Could you check a few things on this model? Use its own coordinates, in mm. Give positions to 0.01 mm unless a question says otherwise; leave off trailing zeros. Order: outer loops, then holes, each group sorted by start corner. A loop starts at its lowest first (then second) coordinate and runs counter-clockwise, first axis right, second up. Notation, with made-up numbers: (83.25, 77.25) -> (115.25, 77.25) arc R25 ccw to (115.25, 107.25) -> close; hole circle Ø5 at (33, 10.25). An arc over 180 degrees is marked (long way). Answer as CSV lines item,"result". Start each with the question number.
(1) I want a section at A-A (x = 0). Please give me the cut outline in (y, z), plus the area to 3 significant figures.
(2) I need wall thicknesses on L1, parallel to Y at x = 0.25, z = 3.25; L2, parallel to X at y = -55, z = 1.75; L3, parallel to Y at x = -1.25, z = -2. Which ranges of each line are inside material? Lowest first, please.
(3) I want a section at C-C (y = -14). Please give me the cut outline in (x, z), plus the area to 3 significant figures.
(4) I want a section at B-B (y = 62.5). Please give me the cut outline in (x, z).
(5) Will these pins go through, and if not, where does the flat tip stop? pin 1 Ø1.4 at (y, z) = (78, 0) entering from -X; pin 2 Ø3 at (y, z) = (38.5, 0) entering from -X; pin 3 Ø1 at (x, y) = (-3, -3) entering from -Z.
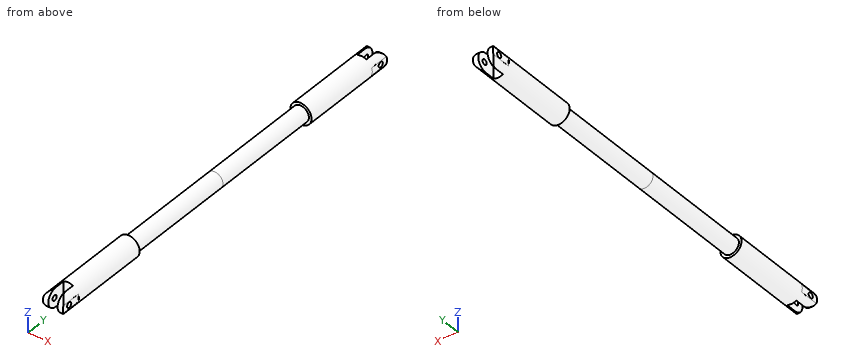
```python
from build123d import *

# Parameters (mm, degrees)
SKETCH2_W               = 3.5
SKETCH2_H               = 22
SKETCH2_W_2             = 3.489149722
SKETCH2_H_2             = 10.808558849
SKETCH2_W_3             = 5.104041679
SKETCH2_H_3             = 8.66936491
CUT_EXTRUDE1_DEPTH      = 10
SKETCH3_R               = 1
CUT_EXTRUDE2_DEPTH      = 1.25
CUT_EXTRUDE2_DEPTH_BACK = 8.75
CUT_EXTRUDE3_DEPTH      = 1.25
CUT_EXTRUDE3_DEPTH_BACK = 8.75


with BuildPart() as part:
    # Sketch1 → Revolve1 (revolve)
    with BuildSketch(Plane.XY, mode=Mode.PRIVATE) as revolve1_sk:
        Polygon((0, -75), (0, 75), (-3, 75), (-3, -35), (-4, -35), (-4, -75), align=None)
    revolve(revolve1_sk.sketch.rotate(Axis((0, -75, 0), (0, 1, 0)), 180), axis=Axis((0, -75, 0), (0, 1, 0)))  # turned: the seam where the file's is

    # Sketch2 → Cut-Extrude1 (cut, symmetric)
    with BuildSketch(Plane.XY):
        with Locations((0, -75)):
            Rectangle(SKETCH2_W, SKETCH2_H)
        with Locations((-5.494574861, -69.404279425)):
            Rectangle(SKETCH2_W_2, SKETCH2_H_2)
        with Locations((6.302020839, -68.334682455)):
            Rectangle(SKETCH2_W_3, SKETCH2_H_3)
    extrude(amount=CUT_EXTRUDE1_DEPTH, both=True, mode=Mode.SUBTRACT)

    # Sketch3 → Cut-Extrude2 (cut, two sides)
    with BuildSketch(Plane(origin=(3.75, 0, 0), x_dir=(0, 0, -1), z_dir=(1, 0, 0))) as cut_extrude2_sk:
        with Locations(Location((0, -68.334682455, 0), (0, 0, 90))):  # turned: the seam where the file's is
            Circle(SKETCH3_R)
    extrude(amount=CUT_EXTRUDE2_DEPTH, mode=Mode.SUBTRACT)
    extrude(cut_extrude2_sk.sketch, amount=-CUT_EXTRUDE2_DEPTH_BACK, mode=Mode.SUBTRACT)

    # Sketch4 → Cut-Extrude3 (cut, two sides)
    with BuildSketch(Plane(origin=(3.75, 0, 0), x_dir=(0, 0, -1), z_dir=(1, 0, 0))) as cut_extrude3_sk:
        with BuildLine():
            Line((-3.596873642, -67.828802158), (-5.675638146, -67.828802158))
            Line((-5.675638146, -67.828802158), (-5.675638146, -76.926900892))
            Line((-5.675638146, -76.926900892), (6.407188639, -76.926900892))
            Line((6.407188639, -76.926900892), (6.407188639, -67.828802158))
            Line((6.407188639, -67.828802158), (3.596873642, -67.828802158))
            ThreePointArc((3.596873642, -67.828802158), (0, -71.334682455), (-3.596873642, -67.828802158))
        make_face()
    extrude(amount=CUT_EXTRUDE3_DEPTH, mode=Mode.SUBTRACT)
    extrude(cut_extrude3_sk.sketch, amount=-CUT_EXTRUDE3_DEPTH_BACK, mode=Mode.SUBTRACT)

    # Split1
    split(bisect_by=Plane.ZX.offset(6), keep=Keep.BOTTOM)

    # Mirror1: part across plane


with BuildPart() as part_1:
    add(part.part)
    add(part.part.mirror(Plane.ZX.offset(6)))


solid = part_1.part
```
Final values:
1,outline,"(-64, -4) -> (-35, -4) -> (-35, -3) -> (47, -3) -> (47, -4) -> (76, -4) -> (76, 4) -> (47, 4) -> (47, 3) -> (-35, 3) -> (-35, 4) -> (-64, 4) -> close"
1,area,"956 mm²"
2,L1,"-64 to -35, 47 to 76"
2,L2,"-3.6 to 3.6"
2,L3,"-64 to 76"
3,outline,"circle Ø6 at (0, 0)"
3,area,"28.3 mm²"
4,outline,"circle Ø8 at (0, 0)"
5,pin 1,"x = -3.75"
5,pin 2,"x = -3"
5,pin 3,"z = -1.66"
